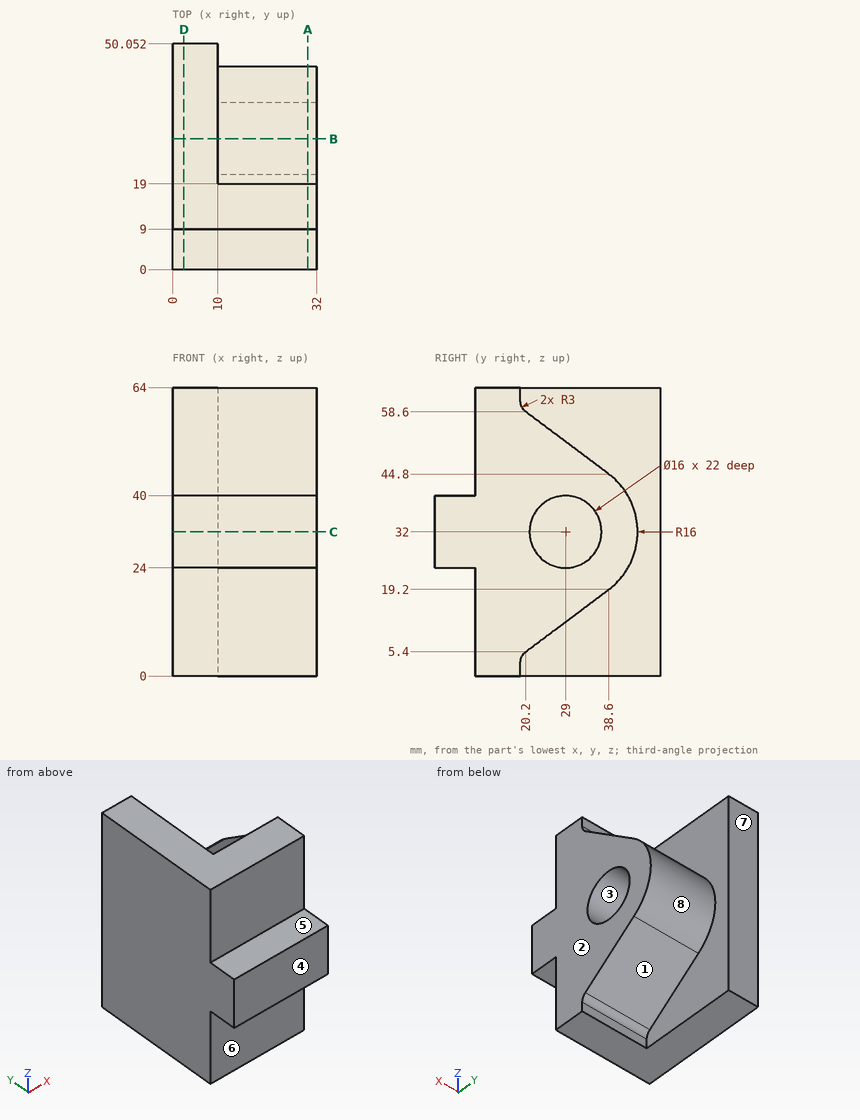
Source: three-view drawing plus pictorial views. Frame: mm from the lowest corner of the part. A direction names the side the tool comes from. Give positions to 0.01 mm unless a question says otherwise; leave off trailing zeros. Write each loop counter-clockwise with the first axis right and the second up, starting at its lowest first coordinate (ties: lowest second). Pieces come first, ordered by that corner, then holes. Notation, with made-up numbers: M -38.75,8 L -21.75,8 A30 cw -21.75,44 Z; hole C -7.75,77 d3. An arc over 180 degrees is marked long. Use one line per item in the form item = value.
1. Mould query, pull axis Z, two halves, no side actions, for the marked faces 1, 2 and 3. Classes: released by +Z, released by -Z, zero draft, split by the parting line, or undercut.
Outcome:
face_1 = released by -Z
face_2 = zero draft
face_3 = undercut
2. Ray query, L1, parallel to Y at x = 17.75, z = 32; L2, parallel to Y at x = 12, z = 6; L3, parallel to X at y = 47, z = 26. Return the intervals inside material, ascending.
Outcome:
L1 = 0 to 21, 37 to 45
L2 = 9 to 21
L3 = 0 to 10
3. Cut plane B-B on y = 29. Return loops of the section in (x, z), and give its area (3 significant figures).
Outcome:
outline = M 0,0 L 10,0 L 10,12 L 32,12 L 32,24 L 10,24 L 10,40 L 32,40 L 32,52 L 10,52 L 10,64 L 0,64 Z
area = 1,170 mm²
4. Cut plane A-A on x = 30. Return loops of the section in (y, z).
Outcome:
outline = M 0,24 L 9,24 L 9,0 L 19,0 L 19,3 A3 cw 20.2,5.4 L 38.6,19.2 A16 ccw 38.6,44.8 L 20.2,58.6 A3 cw 19,61 L 19,64 L 9,64 L 9,40 L 0,40 Z; hole C 29,32 d16
5. First-contact query: P1, Ø19, axis at x = 8.5, z = 6.5, coming from the -Y side; P2, Ø8, axis at x = 26, z = 54.5, coming from the +Y side; P3, Ø1, axis at y = 35.5, z = 35.5, coming from the +X side. Flat tips, straight axial feed; report the tip coordinate or a pass-through.
Outcome:
P1 = 9
P2 = 31
P3 = 10
6. Cut plane C-C on z = 32. Return loops of the section in (x, y), and give its area (3 significant figures).
Outcome:
outline = M 0,0 L 32,0 L 32,21 L 10,21 L 10,37 L 32,37 L 32,45 L 10,45 L 10,50.05 L 0,50.05 Z
area = 1,140 mm²
7. Cut plane D-D on x = 2.5. Return loops of the section in (y, z).
Outcome:
outline = M 0,24 L 9,24 L 9,0 L 50.05,0 L 50.05,64 L 9,64 L 9,40 L 0,40 Z
8. Reachability of the marked faces 4, 5, 6, 7 and 8 from +Z, -Z, +X, -X, +Y, -Y: full face, straight path, thin tool, end or side. Return the list, or none.
Outcome:
face_4 = +Z, -Z, +X, -X, -Y
face_5 = +Z, +X, -X, -Y
face_6 = -Z, +X, -X, -Y
face_7 = +Z, -Z, +X, -X, +Y
face_8 = +X, +Y
